Design review of the part built by this model. Coordinates are the model's own, in mm. Face numbers are marked on the shaded views. Coordinates: 2 decimals unless noted, no trailing zeros. Write each loop counter-clockwise with the first axis right and the second up, starting at its lowest first coordinate (ties: lowest second). Pieces come first, ordered by that corner, then holes.
Q1. Take a section at B-B (x = -1.75). Give the boundary of the cut face in (y, z), and give its area (3 significant figures).
Q2. Take a section at A-A (z = -0.2). Give the boundary of the cut face in (x, y).
Q3. For probe 1 along X at (y, z) = (6.5, -1.15); probe 2 along X at (y, z) = (1.75, 0.85); probe 3 along X at (y, z) = (0.75, -1.05), list the stretches that pass through material, from the lowest coordinate up.
Q4. Insertion check: pin 1 (1.5 mm diameter, centred on x = 3.5, z = 0, fed in from +Y); pin 2 (2.5 mm diameter, centred on x = 7.94, z = -0.35, fed in from -Y). Each pin has a flat end and moves straight along its axis. Give the tip position at first contact, or say it passes through.
Q5. Take a section at D-D (y = 1.75). Give the boundary of the cut face in (x, z) (3 decimals).
Q6. Take a section at C-C (y = 6.25). Give the boundary of the cut face in (x, z) (3 decimals), and give its area (3 significant figures).
Q7. Mouldability with a two-part tool opening along X and no side actions: class the marked faces 1, 2 and 3 as pulls with the +X half, pulls with the -X half, needs draft (parallel to the pull), parting line crosses it, or undercut.
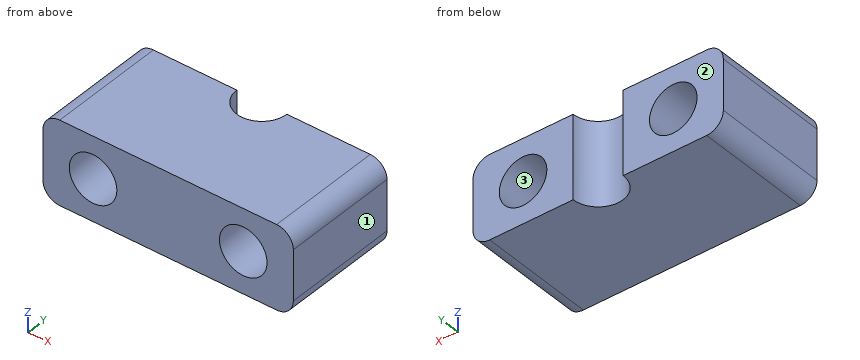
```python
from build123d import *

# Parameters (mm, degrees)
SKETCH1_W           = 15
SKETCH1_H           = 5
BOSS_EXTRUDE1_DEPTH = 7
SKETCH2_R           = 1.5
CUT_EXTRUDE1_DEPTH  = 14.917492532
SKETCH3_R           = 1.425
CUT_EXTRUDE2_DEPTH  = 14.296591966
FILLET1_R           = 1


with BuildPart() as part:
    # Sketch1 → Boss-Extrude1 (new body)
    with BuildSketch(Plane(origin=(0, 0, 0), x_dir=(1, 0, 0), z_dir=(0, 1, 0))):
        with Locations((3.440594059, 0.346534653)):
            Rectangle(SKETCH1_W, SKETCH1_H)
    extrude(amount=BOSS_EXTRUDE1_DEPTH)

    # Sketch2 → Cut-Extrude1 (cut, through all)
    with BuildSketch(Plane(origin=(0, 0, -2.846534653), x_dir=(-1, 0, 0), z_dir=(0, 0, -1))):
        with Locations((-3.440594059, 7)):
            Circle(SKETCH2_R)
    extrude(amount=-CUT_EXTRUDE1_DEPTH, mode=Mode.SUBTRACT)

    # Sketch3 → Cut-Extrude2 (cut, through all)
    with BuildSketch(Plane(origin=(0, 7, 0), x_dir=(1, 0, 0), z_dir=(0, 1, 0))):
        with Locations(Location((7.940594059, 0.346534653, 0), (0, 0, 270))):
            Circle(SKETCH3_R)
        with Locations(Location((-1.059405941, 0.346534653, 0), (0, 0, 270))):
            Circle(SKETCH3_R)
    extrude(amount=-CUT_EXTRUDE2_DEPTH, mode=Mode.SUBTRACT)

    # Fillet1
    fillet1_edges = [part.edges().sort_by_distance(p)[0] for p in [
        (-4.059405941, 3.5, -2.846534653),
        (10.940594059, 3.5, -2.846534653),
        (10.940594059, 3.5, 2.153465347),
        (-4.059405941, 3.5, 2.153465347),
    ]]
    fillet(fillet1_edges, radius=FILLET1_R)


solid = part.part
```
Response:
1. outline: (0, -2.85) - (7, -2.85) - (7, -1.59) - (0, -1.59) - close; (0, 0.9) - (7, 0.9) - (7, 2.15) - (0, 2.15) - close
1. area: 17.5 mm2
2. outline: (-4.06, 0) - (-2.48, 0) - (-2.48, 7) - (-4.06, 7) - close; (0.36, 0) - (6.52, 0) - (6.52, 7) - (4.94, 7) arc R1.5 cw to (1.94, 7) - (0.36, 7) - close; (9.36, 0) - (10.94, 0) - (10.94, 7) - (9.36, 7) - close
3. probe 1: x = -4.06 to -2.24, 0.12 to 2.03, 4.85 to 6.76, 9.12 to 10.94
3. probe 2: x = -4.06 to -1.83, -0.29 to 7.17, 8.71 to 10.94
3. probe 3: x = -4.06 to -2.3, 0.18 to 6.7, 9.18 to 10.94
4. pin 1: stops at y = 5.74
4. pin 2: passes through
5. outline: (-4.059, -1.847) arc R1 ccw to (-3.059, -2.847) - (9.941, -2.847) arc R1 ccw to (10.941, -1.847) - (10.941, 1.153) arc R1 ccw to (9.941, 2.153) - (-3.059, 2.153) arc R1 ccw to (-4.059, 1.153) - close; hole circle Ø2.85 at (-1.059, -0.347); hole circle Ø2.85 at (7.941, -0.347)
6. outline: (-4.059, -1.847) arc R1 ccw to (-3.059, -2.847) - (2.142, -2.847) - (2.142, 2.153) - (-3.059, 2.153) arc R1 ccw to (-4.059, 1.153) - close; (4.74, -2.847) - (9.941, -2.847) arc R1 ccw to (10.941, -1.847) - (10.941, 1.153) arc R1 ccw to (9.941, 2.153) - (4.74, 2.153) - close; hole circle Ø2.85 at (-1.059, -0.347); hole circle Ø2.85 at (7.941, -0.347)
6. area: 48.4 mm2
7. face 1: pulls with the +X half
7. face 2: needs draft
7. face 3: undercut
